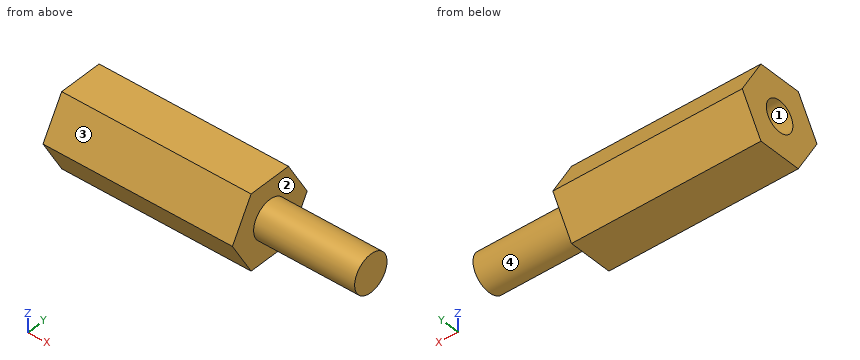
Autodesk Inventor part; units mm, degrees
ref_plane "YZ Plane" through (0, 0, 0) normal (1, 0, 0) x (0, 1, 0)
ref_plane "XZ Plane" through (0, 0, 0) normal (0, 1, 0) x (-1, 0, 0)
ref_plane "XY Plane" through (0, 0, 0) normal (0, 0, 1) x (1, 0, 0)
sketch "スケッチ1" plane through (0, 0, 0) normal (1, 0, 0) x (0, 1, 0)
  line L0 (1.7321, -3) -> (-1.7321, -3)
  line L1 (-1.7321, -3) -> (-3.4641, 0)
  line L2 (-3.4641, 0) -> (-1.7321, 3)
  line L3 (-1.7321, 3) -> (1.7321, 3)
  line L4 (1.7321, 3) -> (3.4641, 0)
  line L5 (3.4641, 0) -> (1.7321, -3)
  point P0 (0, 0)
  point P1 (0, 0)
  dimension "d0" = 6
extrude "押し出し1" add sketch "スケッチ1" along normal blind 15
sketch "スケッチ2" plane through (15, 0, 0) normal (1, 0, 0) x (0, 0, -1)
  circle A0 centre (0, 0) radius 1.5
  dimension "d3" = 3
extrude "押し出し2" add sketch "スケッチ2" along normal blind 8
thread "ねじ1"
sketch "スケッチ3" plane through (0, 0, 0) normal (-1, 0, 0) x (0, 0, 1)
  point P0 (0, 0)
  point P1 (0, 0)
hole "穴1" at (0, 0, 0) direction (1, 0, 0) diameter 2.459 depth 10 tip angle 118
properties part number "Spacer_M3_L15" material "鋼、合金"
For this review, take the finished solid that the model builds, in its own axes (mm). Face numbers are marked on the shaded views. Round coordinates to 2 decimals unless told otherwise and drop trailing zeros. Write each loop counter-clockwise with the first axis right and the second up, starting at its lowest first coordinate (ties: lowest second). Pieces come first, ordered by that corner, then holes. Notation, with made-up numbers: (40, -30) -> (47, -30) arc R22 cw to (47, -19) -> close; hole circle Ø10 at (-31, -35.75). An arc over 180 degrees is marked (long way). Use one line per item in the form item = value.
Q1. Consider section D-D (y = 2.75). State the section outline as (x, z) points.
Resolved:
outline = (0, -1.24) -> (15, -1.24) -> (15, 1.24) -> (0, 1.24) -> close
Q2. Consider section B-B (x = 14.25). State the section outline as (y, z) points, then the cut area to 3 significant figures.
Resolved:
outline = (-3.46, 0) -> (-1.73, -3) -> (1.73, -3) -> (3.46, 0) -> (1.73, 3) -> (-1.73, 3) -> close
area = 31.2 mm²
Q3. Consider section A-A (x = 9.5). State the section outline as (y, z) points, then the cut area to 3 significant figures.
Resolved:
outline = (-3.46, 0) -> (-1.73, -3) -> (1.73, -3) -> (3.46, 0) -> (1.73, 3) -> (-1.73, 3) -> close; hole circle Ø2.46 at (0, 0)
area = 26.4 mm²
Q4. To check wall thickness, follow probe 1 along Z at (x, y) = (5, 0); probe 2 along X at (y, z) = (-2.5, 0.25); probe 3 along Y at (x, z) = (3.5, -0.5). State the ranges of each line that lie inside material, in increasing order. Write a range as from..to.
Resolved:
probe_1 = -3..-1.23, 1.23..3
probe_2 = 0..15
probe_3 = -3.18..-1.12, 1.12..3.18
Q5. Clearance check with flat-ended pins moving along their axes: pin 1 Ø2 at (y, z) = (2, -2) entering from +X; pin 2 Ø2 at (x, z) = (12, 2) entering from -Y; pin 3 Ø2 at (x, y) = (18.5, 0) entering from +Z. State where each tip first meets the part, or that it passes through.
Resolved:
pin_1 = 15
pin_2 = -2.89
pin_3 = 1.5
Q6. The part is to be moulded in two halves that separate along Y. For the marked faces 1, 2, 3 and 4, say which applies: released by +Y, released by -Y, zero draft, split by the parting line, or undercut.
Resolved:
face_1 = undercut
face_2 = zero draft
face_3 = released by -Y
face_4 = split by the parting line
Q7. Consider section C-C (z = 2.4). State the section outline as (x, y) points.
Resolved:
outline = (0, -2.08) -> (15, -2.08) -> (15, 2.08) -> (0, 2.08) -> close
